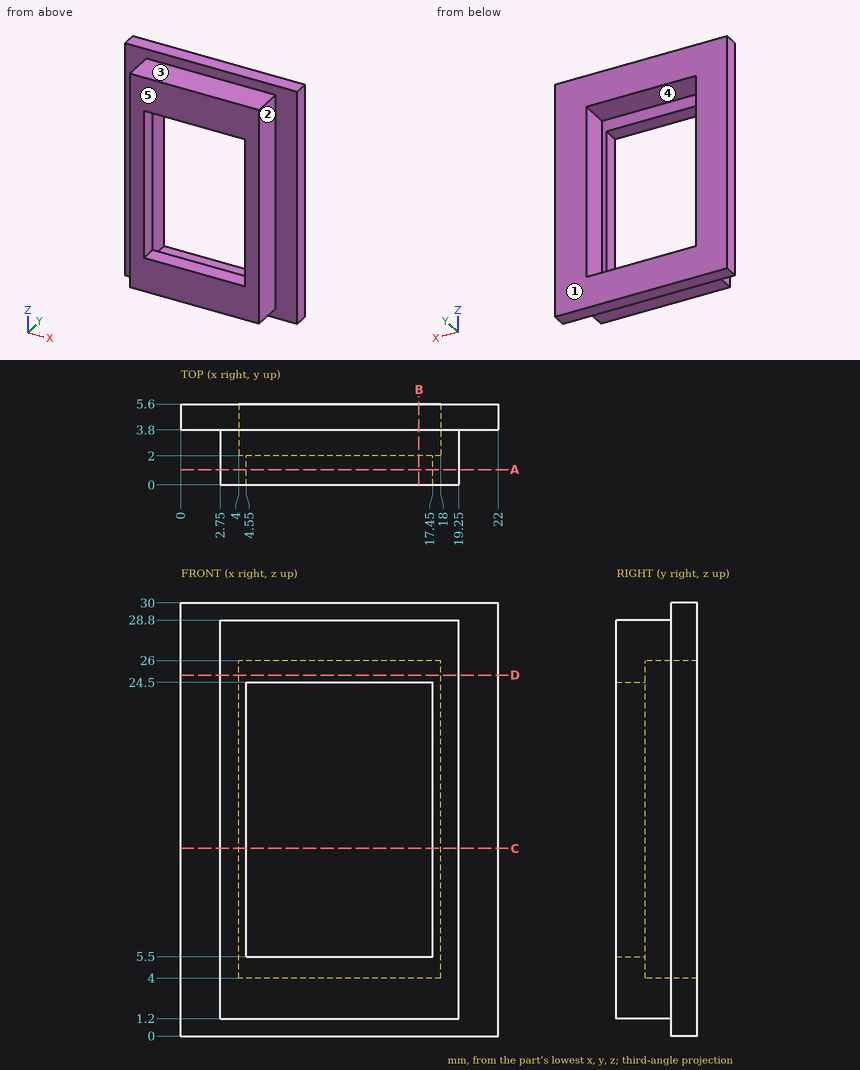
Here's the drawing with two shaded views (mm, measured from the low corner). I have some questions. A direction names the side the tool comes from. Give positions to 0.01 mm unless a question says otherwise; leave off trailing zeros. Loops run counter-clockwise (first coordinate to the right, second up) from the corner with the lowest first, then second, coordinate; pieces in that order, holes last. Notation, with made-up numbers: M 30.5,-32 L 83.5,-32 A7 cw 83.5,-24 Z; hole C -34.5,36.25 d1. An arc over 180 degrees is marked long. One line per item, written item: value. Start each with the question number.
1) On a 3-axis mill with a long thin cutter (end or side, diameter ignored), from which of +Z, -Z, +X, -X, +Y, -Y can I reach the whole of each face in a straight line? I mean the marked faces 1 and 2. Say none if no direction works.
2) If we section it at B-B, the plane x = 16.5: Write out the boundary of the cut face in (y, z), and give its area (3 significant figures).
3) I'm going to push flat-ended pins straight in: pin 1 (1.9 mm diameter, centred on y = 2, z = 11.5, fed in from -X); pin 2 (7 mm diameter, centred on x = 12, z = 10, fed in from +Y); pin 3 (2 mm diameter, centred on y = 1.5, z = 16.5, fed in from +X); pin 4 (2 mm diameter, centred on x = 12, y = 0.5, fed in from +Z). Where does each tip first touch, or does it pass through?
4) If I drill on line 1 (Z direction, x = 8.75, y = 1.9); line 2 (Z direction, x = 16.5, y = 4.3); line 3 (X direction, y = 0.55, z = 22.5), over which ranges is the centre line in solid material (lowest first)? Write a range as [from, to].
5) If we section it at C-C, the plane z = 13: Write out the boundary of the cut face in (x, y), and give its area (3 significant figures).
6) If we section it at D-D, the plane z = 25: Write out the boundary of the cut face in (x, y), and give its area (3 significant figures).
7) If we section it at A-A, the plane y = 1.05: Write out the boundary of the cut face in (x, z).
8) Thinking about a two-plate mould opening in Z: for the marked faces 3, 4 and 5, which applies, +Z half, -Z half, draft (parallel to the pull), parting line (faces both ways), or undercut?
Completed:
1. face 1: +Z, -Z, +X, -X, +Y
1. face 2: +Z, -Z, +X, -Y
2. outline: M 0,1.2 L 3.8,1.2 L 3.8,0 L 5.6,0 L 5.6,4 L 2,4 L 2,5.5 L 0,5.5 Z; M 0,24.5 L 2,24.5 L 2,26 L 5.6,26 L 5.6,30 L 3.8,30 L 3.8,28.8 L 0,28.8 Z
2. area: 41.7 mm^2
3. pin 1: stops at x = 2.75
3. pin 2: passes through
3. pin 3: stops at x = 19.25
3. pin 4: stops at z = 28.8
4. line 1: z = [1.2, 5.5], [24.5, 28.8]
4. line 2: z = [0, 4], [26, 30]
4. line 3: x = [2.75, 4.55], [17.45, 19.25]
5. outline: M 0,3.8 L 2.75,3.8 L 2.75,0 L 4.55,0 L 4.55,2 L 4,2 L 4,5.6 L 0,5.6 Z; M 17.45,0 L 19.25,0 L 19.25,3.8 L 22,3.8 L 22,5.6 L 18,5.6 L 18,2 L 17.45,2 Z
5. area: 26.1 mm^2
6. outline: M 0,3.8 L 2.75,3.8 L 2.75,0 L 19.25,0 L 19.25,3.8 L 22,3.8 L 22,5.6 L 18,5.6 L 18,2 L 4,2 L 4,5.6 L 0,5.6 Z
6. area: 51.9 mm^2
7. outline: M 2.75,1.2 L 19.25,1.2 L 19.25,28.8 L 2.75,28.8 Z; hole M 4.55,5.5 L 17.45,5.5 L 17.45,24.5 L 4.55,24.5 Z
8. face 3: +Z half
8. face 4: undercut
8. face 5: draft
